Solid Edge part; units mm, degrees
sketch "Sketch1" plane through (0, 0, 0) normal (-1, 0, 0) x (0, -1, 0)
  line L0 (25, -17.5) -> (25, 17.5)
  line L1 (25, 17.5) -> (-25, 17.5)
  line L2 (-25, 17.5) -> (-25, -17.5)
  line L3 (-25, -17.5) -> (25, -17.5)
extrude "Protrusion1" add sketch "Sketch1" along normal blind 100
sketch "Sketch2" plane through (-50, 0, 17.5) normal (0, 0, 1) x (0, 1, 0)
  line L0 (20, 45) -> (20, 5)
  line L1 (-20, 5) -> (20, 5)
  line L2 (-20, 45) -> (-20, 5)
  line L3 (-20, 45) -> (20, 45)
extrude "Cutout1" cut sketch "Sketch2" against normal blind 30
sketch "Sketch3" plane through (-105, 10, 2.5) normal (-1, 0, 0) x (0, -1, 0)
  circle A0 centre (0, 0) radius 2.5
  circle A1 centre (20, 0) radius 2.5
extrude "ExtrudedCutout_41" cut sketch "Sketch3" against normal blind 159
fillet "Round_8" radius 2 1 edges at (-50, -25, -17.5)
sketch "Sketch4" plane through (-50, -0.575, -17.5) normal (0, 0, -1) x (0, -1, 0)
  line L0 (-37.0606, 0) -> (53.9819, 0)
  line L1 (41.8981, -54.6569) -> (53.9819, 0)
  line L2 (-28.9495, -54.6569) -> (41.8981, -54.6569)
  line L3 (-37.0606, 0) -> (-28.9495, -54.6569)
  dimension "D1" = 37.0606
extrude "ExtrudedCutout_43" cut sketch "Sketch4" against normal blind 65
sketch "Sketch5" plane through (0, 0, 0) normal (1, 0, 0) x (0, -1, 0)
  line L0 (-25, 11.5) -> (-21.85, 11.5)
  line L1 (-21.85, 11.5) -> (-21.85, 14.65)
  line L2 (-21.85, 14.65) -> (-25, 14.65)
  line L3 (-25, 14.65) -> (-21.85, 17.5)
  line L4 (-21.85, 17.5) -> (-21.85, 20.916)
  line L5 (-21.85, 20.916) -> (-29.169, 20.916)
  line L6 (-29.169, 20.916) -> (-29.169, 11.5)
  line L7 (-29.169, 11.5) -> (-25, 11.5)
extrude "Cutout2" cut sketch "Sketch5" against normal blind 112
sketch "Sketch6" plane through (-50, 0, 0) normal (1, 0, 0) x (0, -1, 0)
  circle A0 centre (-10, -2.5) radius 4.5
  circle A1 centre (10, -2.5) radius 4.5
extrude "ExtrudedProtrusion_35" add sketch "Sketch6" along normal blind 2
chamfer "Chamfer_22" distance 2 angle 45 2 edges at (-48, 14.5, 2.5) (-48, -5.5, 2.5)
sketch "Sketch7" plane through (-100, 0, 0) normal (-1, 0, 0) x (0, 1, 0)
  circle A0 centre (-10, -2.5) radius 4.5
  circle A1 centre (10, -2.5) radius 4.5
extrude "Protrusion2" add sketch "Sketch7" along normal blind 2
chamfer "Chamfer1" distance 2 angle 45 2 edges at (-102, 5.5, 2.5) (-102, -14.5, 2.5)
sketch "Sketch8" plane through (-48, 10, 2.5) normal (1, 0, 0) x (0, -1, 0)
  circle A0 centre (0, 0) radius 2.5
  circle A1 centre (20, 0) radius 2.5
extrude "ExtrudedCutout_46" cut sketch "Sketch8" against normal blind 116
sketch "Sketch9" plane through (-100, 0, 0) normal (-1, 0, 0) x (0, 0, -1)
  line L0 (-17.5, 22) -> (-14.5, 22)
  line L1 (-14.5, 22) -> (-14.5, 19)
  line L2 (-18.2455, 19) -> (-14.5, 19)
  line L3 (-22.1546, 18.9551) -> (-18.2455, 19)
  line L4 (-22.1546, 28.0438) -> (-22.1546, 18.9551)
  line L5 (-14.5, 28.0438) -> (-22.1546, 28.0438)
  line L6 (-14.5, 25) -> (-14.5, 28.0438)
  line L7 (-14.5, 25) -> (-17.5, 22)
extrude "ExtrudedCutout_47" cut sketch "Sketch9" against normal blind 68
Read the model definition and answer for the solid it produces. Units are mm, in the model's axes. A direction names the side the tool comes from. Give positions to 0.01 mm unless a question says otherwise; leave off trailing zeros. Order: outer loops, then holes, each group sorted by start corner. A loop starts at its lowest first (then second) coordinate and runs counter-clockwise, first axis right, second up. Notation, with made-up numbers: (-13.5, 65) -> (16.5, 65) arc R9 ccw to (16.5, 80) -> close; hole circle Ø9 at (-7.75, 48.5). An arc over 180 degrees is marked (long way). Write item = value, one per line.
1. A cutting plane is placed at A-A, the plane x = -53. Write down the section's boundary in (y, z), and give its area (3 significant figures).
Numbers:
outline = (-25, -15.5) arc R2 ccw to (-23, -17.5) -> (21.85, -17.5) -> (25, -14.65) -> (21.85, -14.65) -> (21.85, -11.5) -> (25, -11.5) -> (25, 17.5) -> (-19, 17.5) -> (-19, 14.5) -> (-22, 14.5) -> (-22, 17.5) -> (-25, 14.5) -> close; hole circle Ø5 at (-10, 2.5); hole circle Ø5 at (10, 2.5)
area = 1,680 mm²
2. A cutting plane is placed at C-C, the plane z = -9. Write down the section's boundary in (x, y), and give its area (3 significant figures).
Numbers:
outline = (-100, -25) -> (-50, -25) -> (-50, 25) -> (-100, 25) -> close; hole (-95, -20) -> (-55, -20) -> (-55, 20) -> (-95, 20) -> close
area = 900 mm²
3. The mould has two halves that part along X. Classify faces 1 (the face through (-77, 21, 17.5)), 2 (the face through (-75, 20, 3)): +X half, -X half, draft (parallel to the pull), parting line (faces both ways), or undercut.
Numbers:
face_1 = draft
face_2 = undercut
4. Straight lines are drawn through the part: line 1 along Z through (x, y) = (-99, -10); line 2 along Y through (x, z) = (-97.5, 2.5); line 3 along Y through (x, z) = (-59, -11). For each, find the intervals that lie inside material, in ascending order.
Numbers:
line_1 = -17.5 to 0, 5 to 17.5
line_2 = -25 to -12.5, -7.5 to 7.5, 12.5 to 25
line_3 = -25 to -20, 20 to 25
5. For faces 3 (the face through (-75, -20, 1)), 4 (the face through (-53, -19, 16)), 5 (the face through (-74.6, 23.4, -16.1)), 6 (the face through (-75, 23, -11.5)), determine the directions among +Z, -Z, +X, -X, +Y, -Y from which every point of the face is accessible in a straight line to the end or side of a thin tool.
Numbers:
face_3 = +Z
face_4 = +Z, +X, -X
face_5 = -Z, +X, -X, +Y
face_6 = +X, -X, +Y
6. A cutting plane is placed at D-D, the plane y = -1.5. Write down the section's boundary in (x, z), and give its area (3 significant figures).
Numbers:
outline = (-100, -17.5) -> (-50, -17.5) -> (-50, 17.5) -> (-55, 17.5) -> (-55, -12.5) -> (-95, -12.5) -> (-95, 17.5) -> (-100, 17.5) -> close
area = 550 mm²
7. Given pin 1 (2.5 mm diameter, centred on x = -83, y = -20.5, fed in from +Z); pin 2 (2 mm diameter, centred on y = -4, z = -5.5, fed in from -X); pin 3 (2 mm diameter, centred on y = 17.5, z = -5.5, fed in from +X); pin 4 (4 mm diameter, centred on y = -10, z = 2.5, fed in from -X), each flat-ended and moving along its own axis, determine where each tip first touches the part or whether it passes through.
Numbers:
pin_1 = 14.5
pin_2 = -100
pin_3 = -50
pin_4 = through
8. A cutting plane is placed at B-B, the plane y = 10. Count the separate pieces of the cut face and the enclosed holes in it, and give its area (3 significant figures).
Numbers:
separate_pieces = 3
enclosed_holes = 0
area = 508 mm²
